```python
from build123d import *

# Parameters (mm, degrees)
F1_DEPTH = 94.3654105067
F2_DEPTH = 25.4


with BuildPart() as f1:
    # F0 (on Right) → F1 (new body)
    with BuildSketch(Plane.YZ):
        with BuildLine():
            Line((-39.9835929275, 0), (0, 0))
            Line((0, 0), (34.047730267, 0))
            ThreePointArc((34.047730267, 0), (42.6663665837, 5.9497380049), (40.1583202183, 16.1178242415))
            Line((40.1583202183, 16.1178242415), (-7.4729916735, 58.2961705104))
            ThreePointArc((-7.4729916735, 58.2961705104), (-5.570695265, 55.0765091724), (-4.9089710419, 51.3958744705))
            ThreePointArc((-4.9089710419, 51.3958744705), (-4.9342154485, 50.6658876775), (-5.0098280518, 49.939388722))
            Line((-5.0098280518, 49.939388722), (37.295550108, 12.9483202472))
            ThreePointArc((37.295550108, 12.9483202472), (38.6668473881, 7.4992614051), (34.047730267, 4.2998152785))
            Line((34.047730267, 4.2998152785), (0, 4.2998152785))
            Line((0, 4.2998152785), (-39.9835929275, 4.2998152785))
            Line((-39.9835929275, 4.2998152785), (-39.9835929275, 0))
        make_face()
        with BuildLine():
            ThreePointArc((-4.9089710419, 51.3958744705), (-5.570695265, 55.0765091724), (-7.4729916735, 58.2961705104))
            ThreePointArc((-7.4729916735, 58.2961705104), (-25.6119539634, 48.4083066672), (-5.0098280518, 49.939388722))
            ThreePointArc((-5.0098280518, 49.939388722), (-4.9342154485, 50.6658876775), (-4.9089710419, 51.3958744705))
        make_face()
        with BuildLine():
            ThreePointArc((-9.0356460446, 51.3958744705), (-21.7879990052, 50.1162425544), (-9.5441434252, 53.9041132503))
            ThreePointArc((-9.5441434252, 53.9041132503), (-9.164050414, 52.6755063865), (-9.0356460446, 51.3958744705))
        make_face(mode=Mode.SUBTRACT)
    extrude(amount=F1_DEPTH)

    # F2 (add): a face of the model
    f2_faces = [f1.faces().sort_by_distance(p)[0] for p in [
        (0, -2.9679313302, 1.0377729525),
    ]]
    extrude(f2_faces, amount=F2_DEPTH)


solid = f1.part
```
Check sheet for the modelled part. Datum: model origin and axes. Units: mm. A direction names the side the tool comes from. Give positions to 0.01 mm unless a question says otherwise; leave off trailing zeros. Write each loop counter-clockwise with the first axis right and the second up, starting at its lowest first coordinate (ties: lowest second). Pieces come first, ordered by that corner, then holes. Notation, with made-up numbers: (88.5, -27.75) - (140.5, -27.75) arc R15 ccw to (140.5, -8.75) - close; hole circle Ø8 at (42.25, 50). An arc over 180 degrees is marked (long way). Answer as a JSON object with one key per item and string values. Group by question number.
1) Sectioned sample at D-D (y = 7.5). Record the cut outline in (x, z), then the cut area to 3 significant figures.
2) Sectioned sample at A-A (y = -14). Record the cut outline in (x, z), then the cut area to 3 significant figures.
3) Depth check by flat-ended pin: P1, Ø5, axis at x = 16, z = 15.5, coming from the -Y side; P2, Ø1.5, axis at x = 77.5, z = 44.5, coming from the -Y side; P3, Ø4, axis at x = -6.5, z = 34.5, coming from the +Y side; P4, Ø4, axis at y = 34.5, z = 23, coming from the -X side. Enter the tip coordinate at first touch or a pass-through.
4) Release check for a two-part mould opening along Z. For faces 4 (the face through (35.321, 38.696, 7.578)), 5 (the face through (35, -3, 0)), 6 (the face through (35.32, 16.68, 36.91)) record: pulls with the +Z half, pulls with the -Z half, needs draft (parallel to the pull), parting line crosses it, or undercut.
5) Thickness scan on probe 1 along Z at (x, y) = (79, -14); probe 2 along Z at (x, y) = (39, -30); probe 3 along Z at (x, y) = (55, 26). Record the ranges inside material, lowest first. Write a range as from..to.
6) Sectioned sample at C-C (x = 29.5). Record the cut outline in (y, z), then the cut area to 3 significant figures.
7) Access from +Z, -Z, +X, -X, +Y, -Y to the whole of each face (thin tool, end or side, straight path). Record for faces 1 (the face through (35, -39.984, 2)), 2 (the face through (35, -2, 4.3)), 3 (the face through (35.32, 15.85, 31.7)).
8) Sectioned sample at B-B (z = 43). Record the cut outline in (x, y), then the cut area to 3 significant figures.
Geometry results:
{
 "1": {"outline": "(-25.4, 0) - (94.37, 0) - (94.37, 4.3) - (-25.4, 4.3) - close; (-25.4, 39) - (94.37, 39) - (94.37, 45.04) - (-25.4, 45.04) - close", "area": "1,240 mm^2"},
 "2": {"outline": "(-25.4, 0) - (94.37, 0) - (94.37, 4.3) - (-25.4, 4.3) - close; (-25.4, 40.93) - (94.37, 40.93) - (94.37, 45.13) - (-25.4, 45.13) - close; (-25.4, 57.66) - (94.37, 57.66) - (94.37, 61.86) - (-25.4, 61.86) - close", "area": "1,520 mm^2"},
 "3": {"P1": "stops at y = 31.52", "P2": "stops at y = -24.07", "P3": "stops at y = 21.66", "P4": "stops at x = -25.4"},
 "4": {"face 4": "undercut", "face 5": "pulls with the -Z half", "face 6": "pulls with the +Z half"},
 "5": {"probe 1": "z = 0..4.3, 40.93..45.13, 57.66..61.86", "probe 2": "z = 0..4.3", "probe 3": "z = 0..4.3, 22.82..28.66"},
 "6": {"outline": "(-39.98, 0) - (34.05, 0) arc R9.22 ccw to (40.16, 16.12) - (-7.47, 58.3) arc R10.57 ccw (long way) to (-5.01, 49.94) - (37.3, 12.95) arc R4.93 cw to (34.05, 4.3) - (-39.98, 4.3) - close; hole circle Ø12.88 at (-15.48, 51.4)", "area": "874 mm^2"},
 "7": {"face 1": "+Z, -Z, +X, -X, -Y", "face 2": "+X, -X, -Y", "face 3": "+X, -X"},
 "8": {"outline": "(-25.4, -21.89) - (94.37, -21.89) - (94.37, -9.06) - (-25.4, -9.06) - close; (-25.4, 2.93) - (94.37, 2.93) - (94.37, 9.8) - (-25.4, 9.8) - close", "area": "2,360 mm^2"}
}
